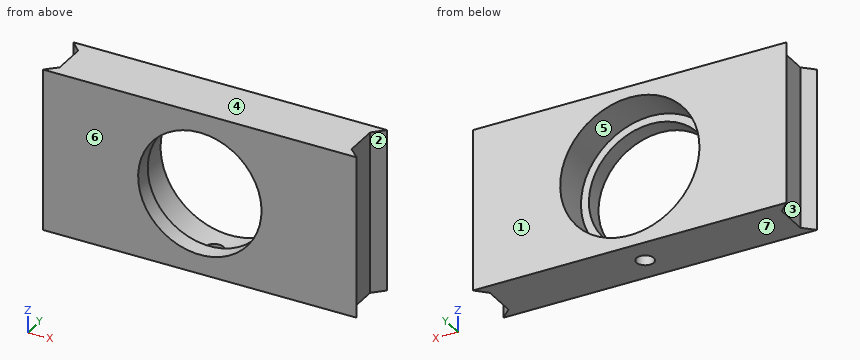
from build123d import *

# Parameters (mm, degrees)
EXTRUDE_1_DEPTH     = 30
SKETCH_2_R          = 11.43
CUT_EXTRUDE_1_DEPTH = 45.733812445
SKETCH_2_3_R        = 12.9
SKETCH_2_3_R_2      = 11.43
CUT_EXTRUDE_2_DEPTH = 6.9
SKETCH_3_R          = 1.6
CUT_EXTRUDE_3_DEPTH = 5


with BuildPart() as part:
    # Sketch 1 → Extrude 1 (new body)
    with BuildSketch(Plane.XY):
        Polygon((29.606806474, -0.652166831), (31.614989733, -2.563983573), (-26.485010267, -2.563983573), (-24.476827008, -0.652166831), (-24.476827008, 5.507833169), (-26.485010267, 7.516016427), (31.614989733, 7.516016427), (29.606806474, 5.507833169), align=None)
    extrude(amount=EXTRUDE_1_DEPTH)

    # Sketch 2 → Cut-Extrude 1 (cut, through all)
    with BuildSketch(Plane(origin=(0, 7.516016427, 0), x_dir=(1, 0, 0), z_dir=(0, 1, 0))):
        with Locations(Location((2.564989733, -15, 0), (0, 0, 270))):
            Circle(SKETCH_2_R)
    extrude(amount=-CUT_EXTRUDE_1_DEPTH, mode=Mode.SUBTRACT)

    # Sketch 2_3 → Cut-Extrude 2 (cut)
    with BuildSketch(Plane(origin=(0, 7.516016427, 0), x_dir=(1, 0, 0), z_dir=(0, 1, 0))):
        with Locations(Location((2.564989733, -15, 0), (0, 0, 270))):
            Circle(SKETCH_2_3_R)
        with Locations(Location((2.564989733, -15, 0), (0, 0, 270))):
            Circle(SKETCH_2_3_R_2, mode=Mode.SUBTRACT)
    extrude(amount=-CUT_EXTRUDE_2_DEPTH, mode=Mode.SUBTRACT)

    # Sketch 3 → Cut-Extrude 3 (cut)
    with BuildSketch(Plane(origin=(0, 0, 0), x_dir=(-1, 0, 0), z_dir=(0, 0, -1))):
        with Locations((-2.556806474, 2.427833169)):
            Circle(SKETCH_3_R)
    extrude(amount=-CUT_EXTRUDE_3_DEPTH, mode=Mode.SUBTRACT)


solid = part.part
Geometry check sheet. Reference: the model listing, model coordinates, mm. Face numbers are marked on the shaded views. A direction names the side the tool comes from. Round coordinates to 2 decimals unless told otherwise and drop trailing zeros. Write each loop counter-clockwise with the first axis right and the second up, starting at its lowest first coordinate (ties: lowest second). Pieces come first, ordered by that corner, then holes. Notation, with made-up numbers: (-21, 53.5) -> (-1, 53.5) arc R11 ccw to (-1, 70.5) -> close; hole circle Ø11 at (43, 48). An arc over 180 degrees is marked (long way). One line per item, written item: value. Start each with the question number.
(1) Cross-section at C-C, the plane y = 3. Record the cut outline in (x, z).
(2) Draft check along Z on the marked faces 4, 5, 6 and 7. Enter one of: +Z half, -Z half, draft (parallel to the pull), parting line (faces both ways), or undercut.
(3) Cross-section at B-B, the plane x = 12. Record the cut outline in (y, z), and give its area (3 significant figures).
(4) Go/stop test with flat-tipped pins: pin 1 Ø1.5 at (y, z) = (0, 18) entering from -X; pin 2 Ø1.8 at (y, z) = (2.5, 15.5) entering from +X; pin 3 Ø1 at (y, z) = (0.5, 12.5) entering from -X. Record where each tip stops, or that it passes through.
(5) Cross-section at A-A, the plane z = 15. Record the cut outline in (x, y), and give its area (3 significant figures).
(6) Scan lines: line 1 (X direction, y = -0.5, z = 14.5); line 2 (X direction, y = 5.5, z = 28.5); line 3 (X direction, y = 5.5, z = 15). Record each from-to range of solid material in increasing order. Write a range as [from, to].
(7) Access from +Z, -Z, +X, -X, +Y, -Y to the whole of each face (thin tool, end or side, straight path). Record for the marked faces 1, 2 and 3.
(8) Cross-section at D-D, the plane y = -1.5. Record the cut outline in (x, z).
Answer:
1. outline: (-24.48, 0) -> (1.06, 0) -> (1.06, 2.19) arc R12.9 cw (long way) to (4.05, 2.19) -> (4.05, 0) -> (29.61, 0) -> (29.61, 30) -> (-24.48, 30) -> close
2. face 4: +Z half
2. face 5: undercut
2. face 6: draft
2. face 7: -Z half
3. outline: (-2.56, 0) -> (7.52, 0) -> (7.52, 6.2) -> (0.62, 6.2) -> (0.62, 8.55) -> (-2.56, 8.55) -> close; (-2.56, 21.45) -> (0.62, 21.45) -> (0.62, 23.8) -> (7.52, 23.8) -> (7.52, 30) -> (-2.56, 30) -> close
3. area: 140 mm²
4. pin 1: x = -24.58
4. pin 2: x = 29.61
4. pin 3: x = -24.48
5. outline: (-26.49, -2.56) -> (-8.87, -2.56) -> (-8.87, 0.62) -> (-10.34, 0.62) -> (-10.34, 7.52) -> (-26.49, 7.52) -> (-24.48, 5.51) -> (-24.48, -0.65) -> close; (13.99, -2.56) -> (31.61, -2.56) -> (29.61, -0.65) -> (29.61, 5.51) -> (31.61, 7.52) -> (15.46, 7.52) -> (15.46, 0.62) -> (13.99, 0.62) -> close
5. area: 302 mm²
6. line 1: [-24.48, -8.85], [13.98, 29.61]
6. line 2: [-24.48, 29.61]
6. line 3: [-24.48, -10.34], [15.46, 29.61]
7. face 1: +Z, -Z, +X, -X, +Y
7. face 2: +Z, -Z, +X
7. face 3: +Z, -Z, -X
8. outline: (-25.37, 0) -> (30.5, 0) -> (30.5, 30) -> (-25.37, 30) -> close; hole circle Ø22.86 at (2.56, 15)
